Geometry: final body of the model. Coordinates: model frame, mm. A direction names the side the tool comes from. Coordinates: 2 decimals unless noted, no trailing zeros. Write each loop counter-clockwise with the first axis right and the second up, starting at its lowest first coordinate (ties: lowest second). Pieces come first, ordered by that corner, then holes. Notation, with made-up numbers: (61.5, 65) - (88.5, 65) arc R21 ccw to (88.5, 99) - close; hole circle Ø3 at (66.5, 45.25). An arc over 180 degrees is marked (long way). Answer as a JSON object with one key per item and string values. Group by question number.
Item 1: Line query: line 1 along X through (y, z) = (3.5, 1.15); line 2 along Y through (x, z) = (3.8, 2.1); line 3 along Y through (x, z) = (31.5, 1). Output: solid intervals per line, ascending. Write a range as from..to.
Item 2: Set-up query: faces 1 (the flat face through (0, 19, 2)), 2 (the cylindrical face through (4.123, 4.006, 1.479)). Return all of +Z, -Z, +X, -X, +Y, -Y with unobstructed straight access to the full face (end or side cutting, diameter ignored); none if empty.
Item 3: Section A-A on x = 41.5. Return loops of the section in (y, z).
Item 4: Section B-B on z = 1. Return loops of the section in (x, y).
Item 5: Section D-D on x = 52.8. Return loops of the section in (y, z).
Item 6: First-contact query: pin 1 Ø4.5 at (x, y) = (3.5, 34) entering from -Z; pin 2 Ø2.5 at (x, y) = (3, 15.5) entering from -Z. Flat tips, straight axial feed; report the tip coordinate or a pass-through.
Item 7: Mould query, pull axis Y, two halves, no side actions, for faces 3 (the flat face through (15, 19, 5)), 4 (the flat face through (51, 19, 3)), 5 (the flat face through (28, 38, 2)). Classes: pulls with the +Y half, pulls with the -Y half, needs draft (parallel to the pull), parting line crosses it, or undercut.
Item 8: Section C-C on y = 25. Return loops of the section in (x, z), and give its area (3 significant figures).
```python
from build123d import *

# Parameters (mm, degrees)
CYLINDER_R       = 0.6
CYLINDER_DEPTH   = 3
ARRAY001_X_COUNT = 2
ARRAY001_X_PITCH = 49
ARRAY001_Y_COUNT = 2
ARRAY001_Y_PITCH = 31
BOX008_W         = 31
BOX008_H         = 30.6
BOX008_DEPTH     = 10
BOX001_W         = 42
BOX001_H         = 36
BOX001_DEPTH     = 4.5
BOX002_W         = 4
BOX002_H         = 4
BOX002_DEPTH     = 2.4
ARRAY_X_COUNT    = 2
ARRAY_X_PITCH    = 50.6
ARRAY_Y_COUNT    = 2
ARRAY_Y_PITCH    = 32
BOX003_W         = 54.6
BOX003_H         = 36
BOX003_DEPTH     = 3.9
FILLET001_R      = 1
BOX_W            = 56.6
BOX_H            = 38
BOX_DEPTH        = 6.5
FILLET_R         = 1


with BuildPart() as hole_array:
    # Cylinder → Cylinder (new body)
    with BuildSketch(Plane(origin=(3.8, 3.5, 0), x_dir=(1, 0, 0), z_dir=(0, 0, 1))):
        Circle(CYLINDER_R)
    extrude(amount=CYLINDER_DEPTH)

    # Array001 X: hole array ×2


with BuildPart() as hole_array_1:
    add(hole_array.part)
    with Locations(*[(i * ARRAY001_X_PITCH, 0, 0) for i in range(1, ARRAY001_X_COUNT)]):
        add(hole_array.part)

    # Array001 Y: hole array ×2


with BuildPart() as hole_array_2:
    add(hole_array_1.part)
    with Locations(*[(0, i * ARRAY001_Y_PITCH, 0) for i in range(1, ARRAY001_Y_COUNT)]):
        add(hole_array_1.part)


with BuildPart() as display_hole:
    # Box008 → Box008 (new body)
    with BuildSketch(Plane(origin=(17.5, 3.7, 0), x_dir=(1, 0, 0), z_dir=(0, 0, 1))):
        with Locations((15.5, 15.3)):
            Rectangle(BOX008_W, BOX008_H)
    extrude(amount=BOX008_DEPTH)


with BuildPart() as hole_fusion:
    # Box001 → Box001 (new body)
    with BuildSketch(Plane(origin=(9, 1, 0), x_dir=(1, 0, 0), z_dir=(0, 0, 1))):
        with Locations((21, 18)):
            Rectangle(BOX001_W, BOX001_H)
    extrude(amount=BOX001_DEPTH)

    # Fusion001: union hole array, display_hole
    add(hole_array_2.part)
    add(display_hole.part)


with BuildPart() as hole_stand_array:
    # Box002 → Box002 (new body)
    with BuildSketch(Plane(origin=(1, 1, 0), x_dir=(1, 0, 0), z_dir=(0, 0, 1))):
        with Locations((2, 2)):
            Rectangle(BOX002_W, BOX002_H)
    extrude(amount=BOX002_DEPTH)

    # Array X: hole stand array ×2


with BuildPart() as hole_stand_array_1:
    add(hole_stand_array.part)
    with Locations(*[(i * ARRAY_X_PITCH, 0, 0) for i in range(1, ARRAY_X_COUNT)]):
        add(hole_stand_array.part)

    # Array Y: hole stand array ×2


with BuildPart() as hole_stand_array_2:
    add(hole_stand_array_1.part)
    with Locations(*[(0, i * ARRAY_Y_PITCH, 0) for i in range(1, ARRAY_Y_COUNT)]):
        add(hole_stand_array_1.part)


with BuildPart() as top_cover_extract_fillet:
    # Box003 → Box003 (new body)
    with BuildSketch(Plane(origin=(1, 1, -1.5), x_dir=(1, 0, 0), z_dir=(0, 0, 1))):
        with Locations((27.3, 18)):
            Rectangle(BOX003_W, BOX003_H)
    extrude(amount=BOX003_DEPTH)

    # Fillet001
    fillet001_edges = [top_cover_extract_fillet.edges().sort_by_distance(p)[0] for p in [
        (1, 1, 0.45),
        (1, 37, 0.45),
        (55.6, 1, 0.45),
        (55.6, 37, 0.45),
    ]]
    fillet(fillet001_edges, radius=FILLET001_R)


with BuildPart() as obj1:
    # Box → Box (new body)
    with BuildSketch(Plane.XY.offset(-1.5)):
        with Locations((28.3, 19)):
            Rectangle(BOX_W, BOX_H)
    extrude(amount=BOX_DEPTH)

    # Fillet
    fillet_edges = [obj1.edges().sort_by_distance(p)[0] for p in [
        (0, 0, 1.75),
        (0, 38, 1.75),
        (56.6, 0, 1.75),
        (56.6, 38, 1.75),
    ]]
    fillet(fillet_edges, radius=FILLET_R)

    # Cut: cut top cover extract fillet
    add(top_cover_extract_fillet.part, mode=Mode.SUBTRACT)

    # Fusion: union hole stand array
    add(hole_stand_array_2.part)

    # Cut001: cut hole fusion
    add(hole_fusion.part, mode=Mode.SUBTRACT)


solid = obj1.part
```
Checks:
{
 "1": {"line 1": "0..3.2, 4.4..5, 51.6..52.2, 53.4..56.6", "line 2": "0..2.9, 4.1..5, 33..33.9, 35.1..38", "line 3": "0..1, 37..38"},
 "2": {"face 1": "+Z, -Z, -X, +Y, -Y", "face 2": "-Z"},
 "3": {"outline": "(0, -1.5) - (1, -1.5) - (1, 4.5) - (3.7, 4.5) - (3.7, 5) - (0, 5) - close; (34.3, 4.5) - (37, 4.5) - (37, -1.5) - (38, -1.5) - (38, 5) - (34.3, 5) - close"},
 "4": {"outline": "(0, 1) arc R1 ccw to (1, 0) - (55.6, 0) arc R1 ccw to (56.6, 1) - (56.6, 37) arc R1 ccw to (55.6, 38) - (1, 38) arc R1 ccw to (0, 37) - close; hole (1, 5) - (5, 5) - (5, 1) - (51.6, 1) - (51.6, 5) - (55.6, 5) - (55.6, 33) - (51.6, 33) - (51.6, 37) - (5, 37) - (5, 33) - (1, 33) - close; hole circle Ø1.2 at (3.8, 3.5); hole circle Ø1.2 at (3.8, 34.5); hole circle Ø1.2 at (52.8, 3.5); hole circle Ø1.2 at (52.8, 34.5)"},
 "5": {"outline": "(0, -1.5) - (1, -1.5) - (1, 0) - (2.9, 0) - (2.9, 3) - (4.1, 3) - (4.1, 0) - (5, 0) - (5, 2.4) - (33, 2.4) - (33, 0) - (33.9, 0) - (33.9, 3) - (35.1, 3) - (35.1, 0) - (37, 0) - (37, -1.5) - (38, -1.5) - (38, 5) - (0, 5) - close"},
 "6": {"pin 1": "z = 0", "pin 2": "z = 2.4"},
 "7": {"face 3": "needs draft", "face 4": "undercut", "face 5": "pulls with the +Y half"},
 "8": {"outline": "(0, -1.5) - (1, -1.5) - (1, 2.4) - (9, 2.4) - (9, 4.5) - (17.5, 4.5) - (17.5, 5) - (0, 5) - close; (48.5, 4.5) - (51, 4.5) - (51, 2.4) - (55.6, 2.4) - (55.6, -1.5) - (56.6, -1.5) - (56.6, 5) - (48.5, 5) - close", "area": "51.3 mm^2"}
}
